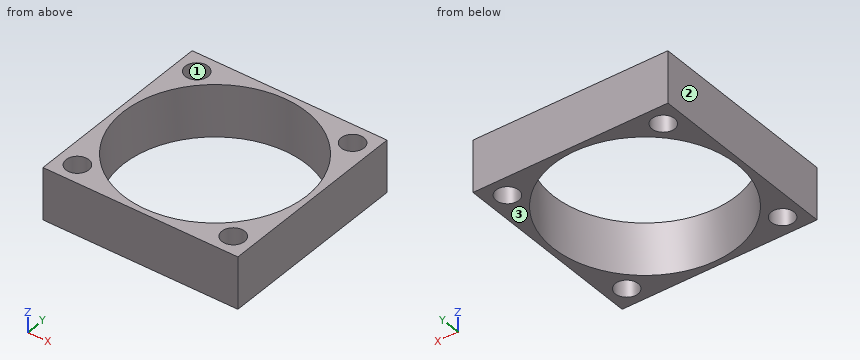
Autodesk Inventor part; units mm, degrees
ref_plane "YZ Plane" through (0, 0, 0) normal (1, 0, 0) x (0, 1, 0)
ref_plane "XZ Plane" through (0, 0, 0) normal (0, 1, 0) x (-1, 0, 0)
ref_plane "XY Plane" through (0, 0, 0) normal (0, 0, 1) x (1, 0, 0)
sketch "Sketch1" plane through (0, 0, 0) normal (0, 0, 1) x (1, 0, 0)
  line L0 (-15, -15) -> (15, -15)
  line L1 (15, -15) -> (15, 15)
  line L2 (15, 15) -> (-15, 15)
  line L3 (-15, 15) -> (-15, -15)
  line L4 (-15, -15) -> (15, 15) construction
  line L5 (15, -15) -> (-15, 15) construction
  circle A0 centre (0, 0) radius 14.125
  line L6 (-12, -12) -> (12, -12) construction
  line L7 (12, -12) -> (12, 12) construction
  line L8 (12, 12) -> (-12, 12) construction
  line L9 (-12, 12) -> (-12, -12) construction
  line L10 (-12, -12) -> (12, 12) construction
  line L11 (12, -12) -> (-12, 12) construction
  dimension "d0" = 30
  dimension "d1" = 28.25
  dimension "d2" = 24
extrude "Extrusion1" add sketch "Sketch1" against normal blind 8
hole "Hole1" at (-12, 12, 0) at (12, 12, 0) at (12, -12, 0) at (-12, -12, 0) direction (0, 0, -1) diameter 3.5 end through all
properties part number "fan"
CAD build for the part. Positions are in the model's coordinates, mm. Face numbers are marked on the shaded views. Round coordinates to 2 decimals unless told otherwise and drop trailing zeros. Order: outer loops, then holes, each group sorted by start corner. A loop starts at its lowest first (then second) coordinate and runs counter-clockwise, first axis right, second up.
Item 1: Saw through at A-A on y = 0. Write the cut outline in (x, z) (3 decimals).
Item 2: Mould opens along X. For the marked faces 1, 2 and 3 say: pulls with the +X half, pulls with the -X half, needs draft (parallel to the pull), parting line crosses it, or undercut.
Item 3: Saw through at C-C on z = -1.5. Write the cut outline in (x, y) (3 decimals).
Item 4: Saw through at D-D on y = 12. Write the cut outline in (x, z), then the cut area to 3 significant figures.
Item 5: Probe line 1 along Y through (x, z) = (-12, -4.25); line 2 along Y through (x, z) = (-2.5, -1.75). List the from-to ranges inside material, lowest first.
Item 6: Pin check, flat tip, straight feed: pin 1 (2 mm diameter, centred on x = -6.5, y = -11, fed in from -Z). Stop position of the tip, or through.
Reported:
1. outline: (-15, -8) - (-14.125, -8) - (-14.125, 0) - (-15, 0) - close; (14.125, -8) - (15, -8) - (15, 0) - (14.125, 0) - close
2. face 1: undercut
2. face 2: pulls with the -X half
2. face 3: needs draft
3. outline: (-15, -15) - (15, -15) - (15, 15) - (-15, 15) - close; hole circle Ø28.25 at (0, 0); hole circle Ø3.5 at (-12, -12); hole circle Ø3.5 at (-12, 12); hole circle Ø3.5 at (12, -12); hole circle Ø3.5 at (12, 12)
4. outline: (-15, -8) - (-13.75, -8) - (-13.75, 0) - (-15, 0) - close; (-10.25, -8) - (-7.45, -8) - (-7.45, 0) - (-10.25, 0) - close; (7.45, -8) - (10.25, -8) - (10.25, 0) - (7.45, 0) - close; (13.75, -8) - (15, -8) - (15, 0) - (13.75, 0) - close
4. area: 64.8 mm2
5. line 1: y = -15 to -13.75, -10.25 to -7.45, 7.45 to 10.25, 13.75 to 15
5. line 2: y = -15 to -13.9, 13.9 to 15
6. pin 1: passes through
